```python
from build123d import *

# Parameters (mm, degrees)
SKETCH1_W               = 178
SKETCH1_H               = 4
SKETCH1_H_2             = 21.844
SKETCH1_R               = 1.7
BOSS_EXTRUDE1_DEPTH     = 4
SKETCH1_3_W             = 178
SKETCH1_3_H             = 4
BOSS_EXTRUDE2_DEPTH     = 116
SKETCH2_W               = 178
SKETCH2_H               = 4
SKETCH2_H_2             = 21.844
SKETCH2_R               = 1.7
BOSS_EXTRUDE3_DEPTH     = 4
FILLET1_R               = 10
SKETCH3_W               = 15
SKETCH3_H               = 15
SKETCH3_R               = 1.7
BOSS_EXTRUDE4_DEPTH     = 4
FILLET2_R               = 10
SKETCH4_R               = 1.7
CUT_EXTRUDE1_DEPTH      = 16
CUT_EXTRUDE1_DEPTH_BACK = 140


with BuildPart() as part:
    # Sketch1 → Boss-Extrude1 (new body)
    with BuildSketch(Plane.XY):
        with Locations((89, -2)):
            Rectangle(SKETCH1_W, SKETCH1_H)
        with Locations((89, 10.922)):
            Rectangle(SKETCH1_W, SKETCH1_H_2)
        with Locations((164, 10.922)):
            Circle(SKETCH1_R, mode=Mode.SUBTRACT)
        with Locations((14, 10.922)):
            Circle(SKETCH1_R, mode=Mode.SUBTRACT)
    extrude(amount=BOSS_EXTRUDE1_DEPTH)

    # Sketch1<3> → Boss-Extrude2 (add)
    with BuildSketch(Plane.XY):
        with Locations((89, -2)):
            Rectangle(SKETCH1_3_W, SKETCH1_3_H)
    extrude(amount=-BOSS_EXTRUDE2_DEPTH)

    # Sketch2 → Boss-Extrude3 (add)
    with BuildSketch(Plane(origin=(0, 0, -116), x_dir=(-1, 0, 0), z_dir=(0, 0, -1))):
        with Locations((-89, -2)):
            Rectangle(SKETCH2_W, SKETCH2_H)
        with Locations((-89, 10.922)):
            Rectangle(SKETCH2_W, SKETCH2_H_2)
        with Locations((-164, 10.922)):
            Circle(SKETCH2_R, mode=Mode.SUBTRACT)
        with Locations((-14, 10.922)):
            Circle(SKETCH2_R, mode=Mode.SUBTRACT)
    extrude(amount=BOSS_EXTRUDE3_DEPTH)

    # Fillet1
    fillet1_edges = [part.edges().sort_by_distance(p)[0] for p in [
        (0, 21.844, 2),
        (178, 21.844, 2),
        (0, 21.844, -118),
        (178, 21.844, -118),
    ]]
    fillet(fillet1_edges, radius=FILLET1_R)

    # Sketch3 → Boss-Extrude4 (add)
    with BuildSketch(Plane.XZ.offset(4)):
        Polygon((42.5, -135), (42.5, -120), (27.5, -120), align=None)
        with Locations((50, -127.5)):
            Rectangle(SKETCH3_W, SKETCH3_H)
        with Locations((50, -127.5)):
            Circle(SKETCH3_R, mode=Mode.SUBTRACT)
        Polygon((72.5, -120), (57.5, -120), (57.5, -135), align=None)
        Polygon((105.5, 4), (120.5, 4), (120.5, 19), align=None)
        with Locations((128, 11.5)):
            Rectangle(SKETCH3_W, SKETCH3_H)
        with Locations((128, 11.5)):
            Circle(SKETCH3_R, mode=Mode.SUBTRACT)
        Polygon((135.5, 19), (135.5, 4), (150.5, 4), align=None)
    extrude(amount=-BOSS_EXTRUDE4_DEPTH)

    # Fillet2
    fillet2_edges = [part.edges().sort_by_distance(p)[0] for p in [
        (120.5, -2, 19),
        (135.5, -2, 19),
        (42.5, -2, -135),
        (57.5, -2, -135),
    ]]
    fillet(fillet2_edges, radius=FILLET2_R)

    # Sketch4 → Cut-Extrude1 (cut, two sides)
    with BuildSketch(Plane(origin=(0, 0, -120), x_dir=(-1, 0, 0), z_dir=(0, 0, -1))) as cut_extrude1_sk:
        with Locations((-164, 10.922)):
            Circle(SKETCH4_R)
        Polygon((-152, 21.844), (-141.078, 10.922), (-36.922, 10.922), (-26, 21.844), align=None)
    extrude(amount=CUT_EXTRUDE1_DEPTH, mode=Mode.SUBTRACT)
    extrude(cut_extrude1_sk.sketch, amount=-CUT_EXTRUDE1_DEPTH_BACK, mode=Mode.SUBTRACT)


solid = part.part
```
Can you work these out from the model? Positions are in its coordinate system, mm. A direction names the side the tool comes from. Round coordinates to 2 decimals unless told otherwise and drop trailing zeros. Loops run counter-clockwise (first coordinate to the right, second up) from the corner with the lowest first, then second, coordinate; pieces in that order, holes last. Notation, with made-up numbers: M -23.75,41.5 L -11.75,41.5 A17 ccw -11.75,62.5 Z; hole C 65.5,-22.5 d6. An arc over 180 degrees is marked long. Answer as a JSON object with one key per item and string values. Group by question number.
Q1. Imagine slicing it at C-C, the plane z = -48. Please give me the cut outline in (x, y), then the cut area to 3 significant figures.
Q2. Imagine slicing it at B-B, the plane x = 24. Please give me the cut outline in (y, z).
Q3. We'd pull the mould along X, two halves only. Please class faces 1 (the flat face through (50, 0, -124)), 2 (the flat face through (90, 10.922, 2)), 3 (the cylindrical face through (57.235, -1.972, -134.218)): +X half, -X half, draft (parallel to the pull), parting line (faces both ways), or undercut.
Q4. Imagine slicing it at D-D, the plane x = 109. Please give me the cut outline in (y, z), then the cut area to 3 significant figures.
Q5. Will these pins go through, and if not, where does the flat tip stop? pin 1 (4.5 mm diameter, centred on x = 46, z = -124, fed in from +Y); pin 2 (5.5 mm diameter, centred on x = 164, y = 10.922, fed in from -Z); pin 3 (5 mm diameter, centred on x = 104, y = 12, fed in from +Z).
Q6. Please list where these lines run through material, in increasing order: L1, parallel to Y at x = 14, z = -117.9; L2, parallel to Z at x = 49, y = 4; L3, parallel to Y at x = 126.5, z = -54.
Q7. Imagine slicing it at A-A, the plane y = 6.5. Please give me the cut outline in (x, z).
Q8. On a 3-axis mill with a long thin cutter (end or side, diameter ignored), from which of +Z, -Z, +X, -X, +Y, -Y can I reach the whole of each face in a straight line? I mean faces 4 (the flat face through (160, 21.844, -118)), 5 (the flat face through (146.615, 16.459, -118.028)), 6 (the flat face through (90, 9, -116)). Say none if no direction works.
Findings:
{
 "1": {"outline": "M 0,-4 L 178,-4 L 178,0 L 0,0 Z", "area": "712 mm2"},
 "2": {"outline": "M -4,-120 L 21.84,-120 L 21.84,-116 L 0,-116 L 0,0 L 21.84,0 L 21.84,4 L -4,4 Z"},
 "3": {"face 1": "draft", "face 2": "undercut", "face 3": "+X half"},
 "4": {"outline": "M -4,-120 L 10.92,-120 L 10.92,-116 L 0,-116 L 0,0 L 10.92,0 L 10.92,4 L 0,4 L 0,7.5 L -4,7.5 Z", "area": "597 mm2"},
 "5": {"pin 1": "stops at y = 0", "pin 2": "stops at z = -120", "pin 3": "stops at z = 4"},
 "6": {"L1": "y = -4 to 9.22, 12.62 to 21.84", "L2": "z = -120 to -116, 0 to 4", "L3": "y = -4 to 0"},
 "7": {"outline": "M 0,-120 L 178,-120 L 178,-116 L 0,-116 Z; M 0,0 L 178,0 L 178,4 L 0,4 Z"},
 "8": {"face 4": "+Z, -Z, +X, -X, +Y", "face 5": "+Z, -Z, +Y", "face 6": "+X, -X, +Y"}
}
